For this review, take the finished solid that the model builds, in its own axes (mm). Give positions to 0.01 mm unless a question says otherwise; leave off trailing zeros. Write each loop counter-clockwise with the first axis right and the second up, starting at its lowest first coordinate (ties: lowest second). Pieces come first, ordered by that corner, then holes. Notation, with made-up numbers: M 37.5,36.5 L 60.5,36.5 A26 cw 60.5,63.5 Z; hole C 43.25,-14 d6. An arc over 180 degrees is marked long. Write item = value, one per line.
```python
from build123d import *

# Parameters (mm, degrees)
F0_R        = 12.55
F1_DEPTH    = 37
F2_R        = 7.5
F3_DEPTH    = 3
F6_DEPTH    = 95
F7_T2_ANGLE = 359.64
F9_R        = 6.25
F10_DEPTH   = 30
F11_W       = 18.3796742931
F11_H       = 70.2870060131
F12_DEPTH   = 2
F13_DEPTH   = 2.5
F14_W       = 9.4460686669
F14_H       = 6.4466400072
F14_H_2     = 5.4794391096
F14_W_2     = 8.6165779212
F14_W_3     = 0.317027705
F15_DEPTH   = 2.5
F16_DEPTH   = 0.8
F17_R       = 5.7074191609
F18_DEPTH   = 28
F19_R       = 11.3
F20_DEPTH   = 32.8
F21_R       = 2
F22_DEPTH   = 32.8


# Not quite as in the source:
# - a fillet or chamfer that OpenCascade refuses, or shapes differently, is made with other operations: its cross-section is extruded or revolved along the edge and cut away or added


with BuildPart() as f1:
    # F0 (on Front) → F1 (new body)
    with BuildSketch(Plane.XZ):
        Circle(F0_R)
    extrude(amount=F1_DEPTH)

    # F2 (on Front) → F3 (join)
    with BuildSketch(Plane.XZ):
        Circle(F2_R)
    extrude(amount=-F3_DEPTH)

    # F4: fillet of radius 10 on 1 edges, made by hand

    # F4_s1 → F4_t2 (revolve, cut)
    with BuildSketch(Plane.XY):
        with BuildLine():
            ThreePointArc((7.5, 0), (4.2315549177, 2.2195444573), (0.3585715715, 3))
            Line((0.3585715715, 3), (7.5, 3))
            Line((7.5, 3), (7.5, 0))
        make_face()
    revolve(axis=Axis((0, 3, 0), (0, -1, 0)), mode=Mode.SUBTRACT)

    # F5 (on Top) → F6 (join)
    with BuildSketch(Plane.XY):
        with BuildLine():
            Line((-12.4928209826, -12.5774559094), (12.6060726016, -12.3417848491))
            ThreePointArc((12.6060726016, -12.3417848491), (-0.0335977446, -2.8508403226), (-12.4928209826, -12.5774559094))
        make_face()
    extrude(amount=F6_DEPTH)

    # F7: fillet of radius 10 on 1 edges, made by hand

    # F7_s1 → F7_t2 (revolve, cut)
    with BuildSketch(Plane(origin=(-0.1101500857, -0.0013803647, 0), x_dir=(0, 0, 1), z_dir=(-0.9999214878, -0.0125306879, 0))):
        with BuildLine():
            ThreePointArc((85, -28.8501313418), (92.0710678119, -25.9211991536), (95, -18.8501313418))
            Line((95, -18.8501313418), (95, -28.8501313418))
            Line((95, -28.8501313418), (85, -28.8501313418))
        make_face()
    revolve(axis=Axis((0.0884629639, -15.8502672786, 95), (0, 0, 1)), revolution_arc=F7_T2_ANGLE, mode=Mode.SUBTRACT)

    # F9 (on offset) → F10 (join)
    with BuildSketch(Plane.XZ.offset(10)):
        with Locations((-0.0335977446, 85)):
            Circle(F9_R)
    extrude(amount=-F10_DEPTH)

    # F11 (on face) → F12 (cut)
    with BuildSketch(Plane(origin=(0.1169867653, -12.4590536081, 0), x_dir=(0.9999559197, 0.0093892853, 0), z_dir=(0.0093892853, -0.9999559197, 0))):
        with Locations((-0.2562315203, 49.8564969935)):
            Rectangle(F11_W, F11_H)
    extrude(amount=-F12_DEPTH, mode=Mode.SUBTRACT)

    # F11 (on face) → F13 (cut)
    with BuildSketch(Plane(origin=(0.1169867653, -12.4590536081, 0), x_dir=(0.9999559197, 0.0093892853, 0), z_dir=(0.0093892853, -0.9999559197, 0))):
        with BuildLine():
            ThreePointArc((8.9336056262, 85), (-0.2562315203, 94.1898371466), (-9.4460686669, 85))
            Line((-9.4460686669, 85), (8.9336056262, 85))
        make_face()
        with Locations((-0.2562315203, 49.8564969935)):
            Rectangle(F11_W, F11_H)
    extrude(amount=-F13_DEPTH, mode=Mode.SUBTRACT)

    # F14 (on face) → F15 (cut)
    with BuildSketch(Plane(origin=(0.0935135522, -9.9591638088, 0), x_dir=(0.9999559197, 0.0093892853, 0), z_dir=(0.0093892853, -0.9999559197, 0))):
        with Locations((-4.7230343334, 17.9363139905)):
            Rectangle(F14_W, F14_H)
        with Locations((-4.7230343334, 24.4199144393)):
            Rectangle(F14_W, F14_H_2)
        with Locations((-4.7230343334, 30.4199144393)):
            Rectangle(F14_W, F14_H_2)
        with Locations((-4.7230343334, 36.4199144393)):
            Rectangle(F14_W, F14_H_2)
        with Locations((-4.7230343334, 42.4199144393)):
            Rectangle(F14_W, F14_H_2)
        with Locations((-4.7230343334, 48.4199144393)):
            Rectangle(F14_W, F14_H_2)
        with Locations((-4.7230343334, 54.4199144393)):
            Rectangle(F14_W, F14_H_2)
        with Locations((-4.7230343334, 60.4199144393)):
            Rectangle(F14_W, F14_H_2)
        with Locations((-4.7230343334, 66.4199144393)):
            Rectangle(F14_W, F14_H_2)
        with Locations((4.6253166656, 66.4199144393)):
            Rectangle(F14_W_2, F14_H_2)
        with Locations((4.6253166656, 60.4199144393)):
            Rectangle(F14_W_2, F14_H_2)
        with Locations((4.6253166656, 54.4199144393)):
            Rectangle(F14_W_2, F14_H_2)
        with Locations((4.6253166656, 48.4199144393)):
            Rectangle(F14_W_2, F14_H_2)
        with Locations((4.6253166656, 42.4199144393)):
            Rectangle(F14_W_2, F14_H_2)
        with Locations((4.6253166656, 36.4199144393)):
            Rectangle(F14_W_2, F14_H_2)
        with Locations((4.6253166656, 30.4199144393)):
            Rectangle(F14_W_2, F14_H_2)
        with Locations((4.6253166656, 24.4199144393)):
            Rectangle(F14_W_2, F14_H_2)
        with Locations((0.1585138525, 17.9363139905)):
            Rectangle(F14_W_3, F14_H)
        with Locations((4.6253166656, 17.9363139905)):
            Rectangle(F14_W_2, F14_H)
    extrude(amount=-F15_DEPTH, mode=Mode.SUBTRACT)

    # F14 (on face) → F16 (cut)
    with BuildSketch(Plane(origin=(0.0935135522, -9.9591638088, 0), x_dir=(0.9999559197, 0.0093892853, 0), z_dir=(0.0093892853, -0.9999559197, 0))):
        with BuildLine():
            Line((-9.4460686669, 85), (-9.4460686669, 69.6801948845))
            Line((-9.4460686669, 69.6801948845), (0, 69.6801948845))
            Line((0, 69.6801948845), (0.317027705, 69.6801948845))
            Line((0.317027705, 69.6801948845), (8.9336056262, 69.6801948845))
            Line((8.9336056262, 69.6801948845), (8.9336056262, 85))
            ThreePointArc((8.9336056262, 85), (-0.2562315203, 94.1898371466), (-9.4460686669, 85))
        make_face()
    extrude(amount=-F16_DEPTH, mode=Mode.SUBTRACT)

    # F17 (on face) → F18 (cut)
    with BuildSketch(Plane.XZ.offset(10)):
        with Locations((0, 84.9810764194)):
            Circle(F17_R)
    extrude(amount=-F18_DEPTH, mode=Mode.SUBTRACT)

    # F19 (on face) → F20 (cut)
    with BuildSketch(Plane.XZ.offset(37)):
        Circle(F19_R)
    extrude(amount=-F20_DEPTH, mode=Mode.SUBTRACT)

    # F21 (on face) → F22 (join)
    with BuildSketch(Plane.XZ.offset(4.2)):
        with Locations((-7.4610639253, 5.4676343242)):
            Circle(F21_R)
        with Locations((-9.1419702041, -1.4095675888)):
            Circle(F21_R)
        with Locations((-5.4676343242, -7.4610639253)):
            Circle(F21_R)
        with Locations((1.4095675888, -9.1419702041)):
            Circle(F21_R)
        with Locations((7.4610639253, -5.4676343242)):
            Circle(F21_R)
        with Locations((9.1419702041, 1.4095675888)):
            Circle(F21_R)
        with Locations((5.4676343242, 7.4610639253)):
            Circle(F21_R)
        with Locations((-1.4095675888, 9.1419702041)):
            Circle(F21_R)
    extrude(amount=F22_DEPTH)


solid = f1.part
```
1. For line 1 along Z through (x, y) = (-6, -25.5); line 2 along Z through (x, y) = (10, -29.5); line 3 along Y through (x, z) = (4.75, 84), list the stretches that pass through material, from the lowest coordinate up. Write a range as from..to.
Responses:
line_1 = -11.02..-9.58, -9.39..-5.53, 4.1..6.83, 9.58..11.02
line_2 = -7.58..-5.26, -0.4..3.22, 5.26..7.58
line_3 = 18..20
2. We need section A-A, the plane y = -31.5. Count the separate pieces of the cut face and the enclosed holes in it, then the cut area to 3 significant figures.
Responses:
separate_pieces = 9
enclosed_holes = 1
area = 194 mm2
3. Insertion check: P1, Ø6, axis at x = 2, y = -19, coming from the -Z side; P2, Ø0.8, axis at x = 6, y = -9, coming from the -Z side; P3, Ø10, axis at x = -4.5, z = 37.5, coming from the +Y side; P4, Ø3, axis at x = 7, y = -4.5, coming from the +Z side. Each pin has a flat end and moves straight along its axis. Give the tip position at first contact, or say it passes through.
Responses:
P1 = -12.55
P2 = -11.23
P3 = -2.85
P4 = 89.77
4. We need section B-B, the plane z = 42. Write out the cut boundary in (x, y), then the cut area to 3 significant figures.
Responses:
outline = M -12.49,-12.58 L -9.33,-12.55 L -9.38,-7.55 L 0.07,-7.46 L 0.09,-9.96 L 0.41,-9.96 L 0.39,-7.46 L 9,-7.38 L 9.05,-12.38 L 12.61,-12.34 A13 ccw Z
area = 87.2 mm2
5. The part is to be moulded in two halves that separate along Z. For faces 1 (the face through (-5, -37, -7)), 2 (the face through (5, -9, 69.16)), say which applies: +Z half, -Z half, draft (parallel to the pull), parting line (faces both ways), or undercut.
Responses:
face_1 = draft
face_2 = undercut
6. We need section C-C, the plane y = 10. Write out the cut boundary in (x, z), then the cut area to 3 significant figures.
Responses:
outline = C -0.03,85 d12.5; hole C 0,84.98 d11.41
area = 20.4 mm2
